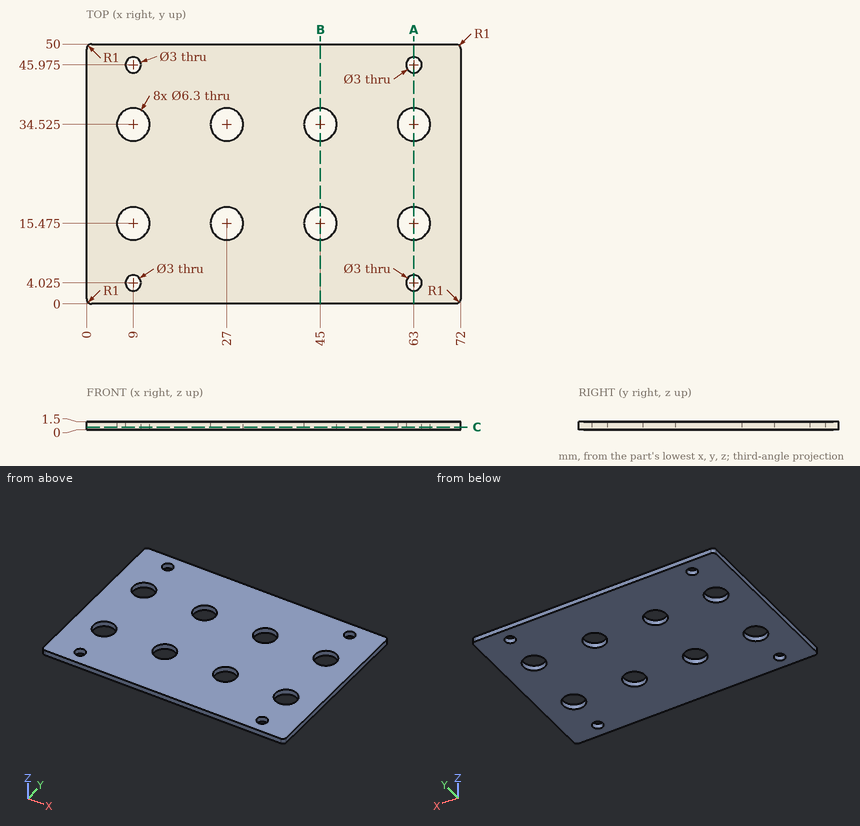
Can you work these out from the drawing? Everything is in mm from the part's minimum corner. Coordinates: 2 decimals unless noted, no trailing zeros. Write each loop counter-clockwise with the first axis right and the second up, starting at its lowest first coordinate (ties: lowest second). Pieces come first, ordered by that corner, then holes. Notation, with made-up numbers: (24, 21.25) - (53, 21.25) arc R14 cw to (53, 40.25) - close; hole circle Ø10 at (79, 44.25). An arc over 180 degrees is marked (long way). Use a Markdown table: item, result.
Q1. Imagine slicing it at B-B (x = 45). List the corners of the cut face in (y, z) for me (3 decimals).
Geometry check:
| item | result |
|---|---|
| outline | (0, 0) - (12.325, 0) - (12.325, 1.5) - (0, 1.5) - close; (18.625, 0) - (31.375, 0) - (31.375, 1.5) - (18.625, 1.5) - close; (37.675, 0) - (50, 0) - (50, 1.5) - (37.675, 1.5) - close |
Q2. Please list where these lines run through material, in increasing order: L1, parallel to Y at x = 63, z = 0.5 (3 decimals); L2, parallel to Y at x = 45, z = 0.4 (3 decimals); L3, parallel to X at y = 5, z = 1.1.
Geometry check:
| item | result |
|---|---|
| L1 | y = 0 to 2.525, 5.525 to 12.325, 18.625 to 31.375, 37.675 to 44.475, 47.475 to 50 |
| L2 | y = 0 to 12.325, 18.625 to 31.375, 37.675 to 50 |
| L3 | x = 0 to 7.86, 10.14 to 61.86, 64.14 to 72 |
Q3. Imagine slicing it at A-A (x = 63). List the corners of the cut face in (y, z) for me (3 decimals), and give its area (3 significant figures).
Geometry check:
| item | result |
|---|---|
| outline | (0, 0) - (2.525, 0) - (2.525, 1.5) - (0, 1.5) - close; (5.525, 0) - (12.325, 0) - (12.325, 1.5) - (5.525, 1.5) - close; (18.625, 0) - (31.375, 0) - (31.375, 1.5) - (18.625, 1.5) - close; (37.675, 0) - (44.475, 0) - (44.475, 1.5) - (37.675, 1.5) - close; (47.475, 0) - (50, 0) - (50, 1.5) - (47.475, 1.5) - close |
| area | 47.1 mm2 |
Q4. Imagine slicing it at C-C (z = 0.5). Count the separate pieces of the cut face and the enclosed holes in it, and give its area (3 significant figures).
Geometry check:
| item | result |
|---|---|
| separate pieces | 1 |
| enclosed holes | 12 |
| area | 3,320 mm2 |
